from build123d import *

# Parameters (mm, degrees)
SKETCH2_R           = 1.4732
SKETCH2_W           = 27.6098
SKETCH2_H           = 57.15
BOSS_EXTRUDE1_DEPTH = 6.0452


with BuildPart() as part:
    # Sketch2 → Boss-Extrude1 (new body)
    with BuildSketch(Plane(origin=(0, 0, 0), x_dir=(1, 0, 0), z_dir=(0, 1, 0))):
        Polygon((-19.05, 34.925), (19.05, 34.925), (19.05, -34.925), (-19.05, -34.925), (-51.9049, -34.925), (-51.9049, 34.925), align=None)
        with Locations(Location((0, 31.75, 0), (0, 0, 90))):
            Circle(SKETCH2_R, mode=Mode.SUBTRACT)
        with Locations(Location((-32.8549, 31.75, 0), (0, 0, 270))):
            Circle(SKETCH2_R, mode=Mode.SUBTRACT)
        with Locations(Location((0, -31.75, 0), (0, 0, 270))):
            Circle(SKETCH2_R, mode=Mode.SUBTRACT)
        with Locations(Location((-32.8549, -31.75, 0), (0, 0, 90))):
            Circle(SKETCH2_R, mode=Mode.SUBTRACT)
        Rectangle(SKETCH2_W, SKETCH2_H, mode=Mode.SUBTRACT)
        with Locations((-32.8549, 0)):
            Rectangle(SKETCH2_W, SKETCH2_H, mode=Mode.SUBTRACT)
    extrude(amount=BOSS_EXTRUDE1_DEPTH)


solid = part.part
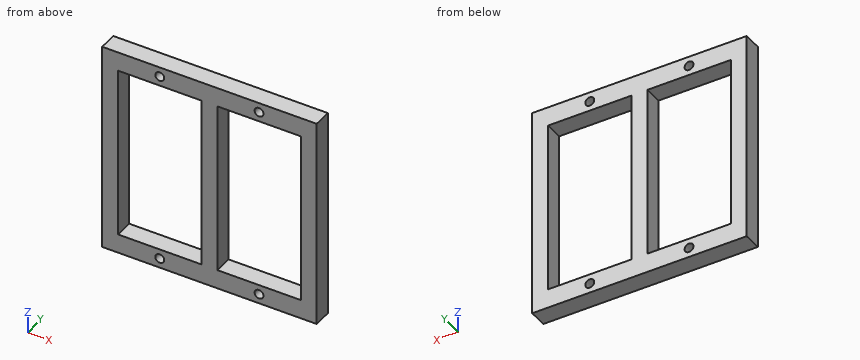
The listing builds one solid part. Answer for the finished solid, in the listing's coordinates (mm). Give positions to 0.01 mm unless a question says otherwise; leave off trailing zeros. Loops run counter-clockwise (first coordinate to the right, second up) from the corner with the lowest first, then second, coordinate; pieces in that order, holes last. Notation, with made-up numbers: (68, -26.5) - (97, -26.5) arc R26 cw to (97, -4.5) - close; hole circle Ø4 at (10.25, -12.75). An arc over 180 degrees is marked (long way). Write each question's results on one line, items separated by ' | '.
1. Find section D-D, the plane y = 3. Write down the section's boundary in (x, z) (3 decimals).
Resolved:
outline: (-51.905, -34.925) - (19.05, -34.925) - (19.05, 34.925) - (-51.905, 34.925) - close; hole (-46.66, -28.575) - (-19.05, -28.575) - (-19.05, 28.575) - (-46.66, 28.575) - close; hole circle Ø2.946 at (-32.855, -31.75); hole circle Ø2.946 at (-32.855, 31.75); hole (-13.805, -28.575) - (13.805, -28.575) - (13.805, 28.575) - (-13.805, 28.575) - close; hole circle Ø2.946 at (0, -31.75); hole circle Ø2.946 at (0, 31.75)
2. Find section B-B, the plane z = -31.75. Write down the section's boundary in (x, y).
Resolved:
outline: (-51.9, 0) - (-34.33, 0) - (-34.33, 6.05) - (-51.9, 6.05) - close; (-31.38, 0) - (-1.47, 0) - (-1.47, 6.05) - (-31.38, 6.05) - close; (1.47, 0) - (19.05, 0) - (19.05, 6.05) - (1.47, 6.05) - close
3. Consider probe 1 along X at (y, z) = (2, 31.75); probe 2 along X at (y, z) = (3, -10); probe 3 along Z at (x, y) = (-38, 0.5) (3 decimals). Determine where each line is inside the solid, lowest interval first. Write a range as from..to.
Resolved:
probe 1: x = -51.9..-34.33, -31.38..-1.47, 1.47..19.05 | probe 2: x = -51.9..-46.66, -19.05..-13.8, 13.8..19.05 | probe 3: z = -34.925..-28.575, 28.575..34.925
4. Find section A-A, the plane x = 0. Write down the section's boundary in (y, z) (3 decimals).
Resolved:
outline: (0, -34.925) - (6.045, -34.925) - (6.045, -33.223) - (0, -33.223) - close; (0, -30.277) - (6.045, -30.277) - (6.045, -28.575) - (0, -28.575) - close; (0, 28.575) - (6.045, 28.575) - (6.045, 30.277) - (0, 30.277) - close; (0, 33.223) - (6.045, 33.223) - (6.045, 34.925) - (0, 34.925) - close
5. Find section C-C, the plane x = -22. Write down the section's boundary in (y, z) (3 decimals), then the cut area to 3 significant figures.
Resolved:
outline: (0, -34.925) - (6.045, -34.925) - (6.045, -28.575) - (0, -28.575) - close; (0, 28.575) - (6.045, 28.575) - (6.045, 34.925) - (0, 34.925) - close | area: 76.8 mm^2
